from build123d import *

# Parameters (mm, degrees)
F0_W      = 508
F0_H      = 508
F1_DEPTH  = 508
F2_R      = 44.45
F3_DEPTH  = 25.4
F4_R      = 44.45
F5_DEPTH  = 25.4
F6_R      = 44.45
F7_DEPTH  = 25.4
F8_R      = 44.45
F9_DEPTH  = 25.4
F10_R     = 44.45
F11_DEPTH = 25.4
F12_R     = 44.45
F13_DEPTH = 25.4


with BuildPart() as f1:
    # F0 (on Top) → F1 (new body)
    with BuildSketch(Plane.XY):
        with Locations((46.919354, 44.886551)):
            Rectangle(F0_W, F0_H)
    extrude(amount=F1_DEPTH)

    # F2 (on face) → F3 (cut)
    with BuildSketch(Plane(origin=(-207.080646, 0, 0), x_dir=(0, -1, 0), z_dir=(-1, 0, 0))):
        with Locations((-171.886551, 127)):
            Circle(F2_R)
        with Locations((-171.886551, 381)):
            Circle(F2_R)
        with Locations((82.113449, 381)):
            Circle(F2_R)
        with Locations((82.113449, 127)):
            Circle(F2_R)
    extrude(amount=-F3_DEPTH, mode=Mode.SUBTRACT)

    # F4 (on face) → F5 (cut)
    with BuildSketch(Plane(origin=(0, 0, 0), x_dir=(1, 0, 0), z_dir=(0, 0, -1))):
        with Locations((-80.080646, 101.163449)):
            Circle(F4_R)
        with Locations((-80.080646, -190.936551)):
            Circle(F4_R)
        with Locations((173.919354, 101.163449)):
            Circle(F4_R)
        with Locations((-80.080646, -44.886551)):
            Circle(F4_R)
        with Locations((173.919354, -44.886551)):
            Circle(F4_R)
        with Locations((173.919354, -190.936551)):
            Circle(F4_R)
    extrude(amount=-F5_DEPTH, mode=Mode.SUBTRACT)

    # F6 (on face) → F7 (cut)
    with BuildSketch(Plane(origin=(0, 298.886551, 0), x_dir=(-1, 0, 0), z_dir=(0, 1, 0))):
        with Locations((80.080646, 127)):
            Circle(F6_R)
        with Locations((-173.919354, 381)):
            Circle(F6_R)
        with Locations((-46.919354, 254)):
            Circle(F6_R)
    extrude(amount=-F7_DEPTH, mode=Mode.SUBTRACT)

    # F8 (on face) → F9 (cut)
    with BuildSketch(Plane.XZ.offset(209.113449)):
        with Locations((-80.080646, 127)):
            Circle(F8_R)
        with Locations((-80.080646, 381)):
            Circle(F8_R)
        with Locations((46.919354, 254)):
            Circle(F8_R)
        with Locations((173.919354, 127)):
            Circle(F8_R)
        with Locations((173.919354, 381)):
            Circle(F8_R)
    extrude(amount=-F9_DEPTH, mode=Mode.SUBTRACT)

    # F10 (on face) → F11 (cut)
    with BuildSketch(Plane.YZ.offset(300.919354)):
        with Locations((44.886551, 254)):
            Circle(F10_R)
    extrude(amount=-F11_DEPTH, mode=Mode.SUBTRACT)

    # F12 (on face) → F13 (cut)
    with BuildSketch(Plane.XY.offset(508)):
        with Locations((173.919354, -82.113449)):
            Circle(F12_R)
        with Locations((-80.080646, 171.886551)):
            Circle(F12_R)
    extrude(amount=-F13_DEPTH, mode=Mode.SUBTRACT)


solid = f1.part
Geometry check sheet. Reference: the model listing, model coordinates, mm. A direction names the side the tool comes from. Give positions to 0.01 mm unless a question says otherwise; leave off trailing zeros. Order: outer loops, then holes, each group sorted by start corner. A loop starts at its lowest first (then second) coordinate and runs counter-clockwise, first axis right, second up.
1. Access from +Z, -Z, +X, -X, +Y, -Y to the whole of each face (thin tool, end or side, straight path). Record for faces 1 (the face through (288.4, 39.1, 298.07)), 2 (the face through (48, 273.487, 255)), 3 (the face through (173, -102, 25.4)).
Completed:
face 1: +X
face 2: +Y
face 3: -Z
2. Draft check along X on faces 4 (the face through (43, 48, 508)), 5 (the face through (-181.681, 173, 128)), 6 (the face through (46, -183.713, 255)). Enter one of: pulls with the +X half, pulls with the -X half, needs draft (parallel to the pull), parting line crosses it, or undercut.
Completed:
face 4: needs draft
face 5: pulls with the -X half
face 6: undercut
3. Scan lines: line 1 (Y direction, x = -108.5, z = 145); line 2 (X direction, y = -132.5, z = 22.5); line 3 (Z direction, x = -84.5, y = 130.5). Record each from-to range of solid material in increasing order.
Completed:
line 1: y = -183.71 to 273.49
line 2: x = -207.08 to -111.61, -48.56 to 142.39, 205.44 to 300.92
line 3: z = 0 to 482.6
4. Sectioned sample at A-A (z = 254). Record the boundary of the cut face in (x, y), then the cut area to 3 significant figures.
Completed:
outline: (-207.08, -209.11) - (2.47, -209.11) - (2.47, -183.71) - (91.37, -183.71) - (91.37, -209.11) - (300.92, -209.11) - (300.92, 0.44) - (275.52, 0.44) - (275.52, 89.34) - (300.92, 89.34) - (300.92, 298.89) - (91.37, 298.89) - (91.37, 273.49) - (2.47, 273.49) - (2.47, 298.89) - (-207.08, 298.89) - close
area: 251,000 mm2
5. Depth check by flat-ended pin: pin 1 (5 mm diameter, centred on x = -72.5, z = 385, fed in from -Y). Enter the tip coordinate at first touch or a pass-through.
Completed:
pin 1: stops at y = -183.71
6. Sectioned sample at C-C (z = 140). Record the boundary of the cut face in (x, y).
Completed:
outline: (-207.08, -209.11) - (-122.59, -209.11) - (-122.59, -183.71) - (-37.57, -183.71) - (-37.57, -209.11) - (131.41, -209.11) - (131.41, -183.71) - (216.43, -183.71) - (216.43, -209.11) - (300.92, -209.11) - (300.92, 298.89) - (-37.57, 298.89) - (-37.57, 273.49) - (-122.59, 273.49) - (-122.59, 298.89) - (-207.08, 298.89) - (-207.08, 214.39) - (-181.68, 214.39) - (-181.68, 129.38) - (-207.08, 129.38) - (-207.08, -39.61) - (-181.68, -39.61) - (-181.68, -124.62) - (-207.08, -124.62) - close
